Part model, mm, in its own coordinate system. A direction names the side the tool comes from. Coordinates: 2 decimals unless noted, no trailing zeros. Write each loop counter-clockwise with the first axis right and the second up, starting at its lowest first coordinate (ties: lowest second). Pieces come first, ordered by that corner, then holes. Notation, with made-up numbers: (68.25, 50.25) -> (76.25, 50.25) arc R17 cw to (76.25, 81.25) -> close; hole circle Ø10 at (-1.5, 45.25). An arc over 180 degrees is marked (long way). Write item = value, one per line.
from build123d import *

# Parameters (mm, degrees)
F0_W     = 63.49
F0_H     = 5
F1_DEPTH = 22.3
F2_W     = 40
F2_H     = 2
F3_DEPTH = 3
F5_DEPTH = 10
F6_R     = 5
F7_W     = 13.3
F7_H     = 20
F8_DEPTH = 25


with BuildPart() as f1:
    # F0 (on Right) → F1 (new body)
    with BuildSketch(Plane.YZ):
        with Locations((0, 2.5)):
            Rectangle(F0_W, F0_H)
    extrude(amount=-F1_DEPTH)

    # F2 (on face) → F3 (join)
    with BuildSketch(Plane.YZ):
        with Locations((0, 2.5)):
            Rectangle(F2_W, F2_H)
    extrude(amount=F3_DEPTH)

    # F4 (on face) → F5 (join)
    with BuildSketch(Plane(origin=(0, 0, 0), x_dir=(1, 0, 0), z_dir=(0, 0, -1))):
        Polygon((0, 30.245), (0, 31.745), (-22.3, 31.745), (-22.3, -31.745), (0, -31.745), (0, -30.245), (-20.8, -30.245), (-20.8, 30.245), align=None)
    extrude(amount=F5_DEPTH)

    # F6
    f6_edges = [f1.edges().sort_by_distance(p)[0] for p in [
        (-22.3, -31.745, -2.5),
        (-22.3, 31.745, -2.5),
        (-20.8, 30.245, -5),
        (-20.8, -30.245, -5),
    ]]
    fillet(f6_edges, radius=F6_R)

    # F7 (on face) → F8 (cut)
    with BuildSketch(Plane(origin=(0, 0, 0), x_dir=(1, 0, 0), z_dir=(0, 0, -1))):
        with Locations((-11.65, 0)):
            Rectangle(F7_W, F7_H)
        Polygon((-18.3, 14), (-5, 14), (-5, 27.745), (-15.8, 27.745), (-18.3, 25.245), align=None)
        Polygon((-5, -27.745), (-5, -14), (-18.3, -14), (-18.3, -25.245), (-15.8, -27.745), align=None)
    extrude(amount=-F8_DEPTH, mode=Mode.SUBTRACT)


solid = f1.part
Q1. Saw through at D-D on x = -1.25. Give the cut face in (y, z) (3 decimals), and give its area (3 significant figures).
Model answer:
outline = (-31.745, -10) -> (-30.245, -10) -> (-30.245, 0) -> (30.245, 0) -> (30.245, -10) -> (31.745, -10) -> (31.745, 5) -> (-31.745, 5) -> close
area = 347 mm²
Q2. Pin check, flat tips, straight feed: pin 1 (12 mm diameter, centred on x = -14, y = 20, fed in from -Z); pin 2 (0.6 mm diameter, centred on x = 1, z = 2, fed in from +Y); pin 3 (0.6 mm diameter, centred on x = 2, z = 3, fed in from -Y). Stop position of each tip, or through.
Model answer:
pin_1 = 0
pin_2 = 20
pin_3 = -20
Q3. Probe line 1 (Y direction, x = -8, z = 3.25) (3 decimals); line 2 (Y direction, x = -8.5, z = -3.5) (3 decimals); line 3 (Y direction, x = -16, z = 0.25) (3 decimals). List the from-to ranges inside material, lowest first. Write a range as from..to.
Model answer:
line_1 = -31.745..-27.745, -14..-10, 10..14, 27.745..31.745
line_2 = -31.745..-30.245, 30.245..31.745
line_3 = -31.745..-27.545, -14..-10, 10..14, 27.545..31.745
Q4. Which spindle directions (+Z, -Z, +X, -X, +Y, -Y) get a long thin tool onto all of the face, cutting with end or side? Do faces 5 (the face through (-18.3, 20, 2)), 6 (the face through (-21, -2, -10)), 7 (the face through (1, 0, 3.5)), 8 (the face through (-8, 30.245, -5)). Say none if no direction does.
Model answer:
face_5 = +Z, -Z
face_6 = -Z, +X, -X, +Y, -Y
face_7 = +Z, +X, +Y, -Y
face_8 = -Z, +X
Q5. Mould opens along Y. For faces 1 (the face through (-3, 0, 0)), 2 (the face through (0, 0, 1)), 3 (the face through (-9, 31.745, -3)), 4 (the face through (-5, 0, 2)) say: released by +Y, released by -Y, zero draft, split by the parting line, or undercut.
Model answer:
face_1 = undercut
face_2 = zero draft
face_3 = released by +Y
face_4 = undercut
Q6. Saw through at C-C on z = 2.75. Give the cut face in (x, y) (3 decimals), and give its area (3 significant figures).
Model answer:
outline = (-22.3, -26.745) arc R5 ccw to (-17.3, -31.745) -> (0, -31.745) -> (0, -20) -> (3, -20) -> (3, 20) -> (0, 20) -> (0, 31.745) -> (-17.3, 31.745) arc R5 ccw to (-22.3, 26.745) -> close; hole (-18.3, -25.245) -> (-15.8, -27.745) -> (-5, -27.745) -> (-5, -14) -> (-18.3, -14) -> close; hole (-18.3, -10) -> (-5, -10) -> (-5, 10) -> (-18.3, 10) -> close; hole (-18.3, 14) -> (-5, 14) -> (-5, 27.745) -> (-15.8, 27.745) -> (-18.3, 25.245) -> close
area = 900 mm²
Q7. Saw through at A-A on y = 23.5. Give the cut face in (x, z).
Model answer:
outline = (-22.3, -10) -> (-20.8, -10) -> (-20.8, 0) -> (-18.3, 0) -> (-18.3, 5) -> (-22.3, 5) -> close; (-5, 0) -> (0, 0) -> (0, 5) -> (-5, 5) -> close
Q8. Saw through at B-B on x = -13.25. Give the cut face in (y, z) (3 decimals).
Model answer:
outline = (-31.745, -10) -> (-30.245, -10) -> (-30.245, 0) -> (-27.745, 0) -> (-27.745, 5) -> (-31.745, 5) -> close; (-14, 0) -> (-10, 0) -> (-10, 5) -> (-14, 5) -> close; (10, 0) -> (14, 0) -> (14, 5) -> (10, 5) -> close; (27.745, 0) -> (30.245, 0) -> (30.245, -10) -> (31.745, -10) -> (31.745, 5) -> (27.745, 5) -> close
